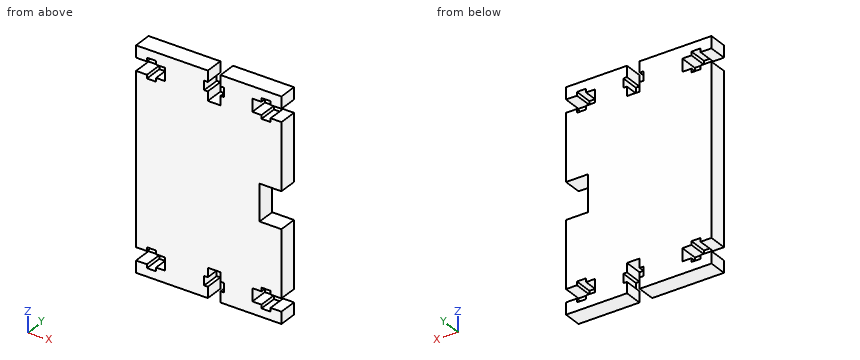
```python
from build123d import *

# Parameters (mm, degrees)
EXTRUDE_1_DEPTH     = 5
CUT_EXTRUDE_1_DEPTH = 5


with BuildPart() as part:
    # 草图1 → 凸台-拉伸1 (new body)
    with BuildSketch(Plane(origin=(0, 0, 0), x_dir=(1, 0, 0), z_dir=(0, 1, 0))):
        Polygon((-19.743275532, 30), (-19.743275532, 26.75), (-16.743275532, 26.75), (-16.743275532, 27.75), (-14.243275532, 27.75), (-14.243275532, 26.75), (-11.743275532, 26.75), (-11.743275532, 23.25), (-14.243275532, 23.25), (-14.243275532, 22.25), (-16.743275532, 22.25), (-16.743275532, 23.25), (-19.743275532, 23.25), (-19.743275532, -23.25), (-16.743275532, -23.25), (-16.743275532, -22.25), (-14.243275532, -22.25), (-14.243275532, -23.25), (-11.743275532, -23.25), (-11.743275532, -26.75), (-14.243275532, -26.75), (-14.243275532, -27.75), (-16.743275532, -27.75), (-16.743275532, -26.75), (-19.743275532, -26.75), (-19.743275532, -30), (20.256724468, -30), (20.256724468, -26.75), (17.256724468, -26.75), (17.256724468, -27.75), (14.756724468, -27.75), (14.756724468, -26.75), (12.256724468, -26.75), (12.256724468, -23.25), (14.756724468, -23.25), (14.756724468, -22.25), (17.256724468, -22.25), (17.256724468, -23.25), (20.256724468, -23.25), (20.256724468, -5), (14.256724468, -5), (14.256724468, 5), (20.256724468, 5), (20.256724468, 23.25), (17.256724468, 23.25), (17.256724468, 22.25), (14.756724468, 22.25), (14.756724468, 23.25), (12.256724468, 23.25), (12.256724468, 26.75), (14.756724468, 26.75), (14.756724468, 27.75), (17.256724468, 27.75), (17.256724468, 26.75), (20.256724468, 26.75), (20.256724468, 30), align=None)
    extrude(amount=EXTRUDE_1_DEPTH)

    # 草图2 → 切除-拉伸1 (cut)
    with BuildSketch(Plane(origin=(0, 5, 0), x_dir=(1, 0, 0), z_dir=(0, 1, 0))):
        Polygon((0, 30), (0, 27), (-1, 27), (-1, 24.5), (0, 24.5), (0, 22), (3.5, 22), (3.5, 24.5), (4.5, 24.5), (4.5, 27), (3.5, 27), (3.5, 30), align=None)
        Polygon((3.5, -30), (0, -30), (0, -27), (-1, -27), (-1, -24.5), (0, -24.5), (0, -22), (3.5, -22), (3.5, -24.5), (4.5, -24.5), (4.5, -27), (3.5, -27), align=None)
    extrude(amount=-CUT_EXTRUDE_1_DEPTH, mode=Mode.SUBTRACT)


solid = part.part
```
Design review of the part built by this model. Coordinates are the model's own, in mm. Give positions to 0.01 mm unless a question says otherwise; leave off trailing zeros. Order: outer loops, then holes, each group sorted by start corner. A loop starts at its lowest first (then second) coordinate and runs counter-clockwise, first axis right, second up. Notation, with made-up numbers: M 89,43.5 L 142,43.5 A15 ccw 142,53.5 Z; hole C 39.5,40 d6. An arc over 180 degrees is marked long. One line per question, with ' | ' between items. Start each with the question number.
Q1. For pin 1 Ø3 at (y, z) = (3, -25) entering from -X; pin 2 Ø0.8 at (y, z) = (3.5, 25) entering from +X, all flat-tipped, find the tip position at first contact; note any pin that passes through.
Q2. We need section A-A (z = 3.5). Write out the cut boundary in (x, y), plus the area to 3 significant figures.
Q3. For L1, parallel to Z at x = -15, y = 2.2; L2, parallel to Z at x = 16, y = 4.55; L3, parallel to X at y = 2.2, z = -23, list the stretches that pass through material, from the lowest coordinate up. Write a range as [from, to].
Returned:
1) pin 1: x = -11.74 | pin 2: x = 12.26
2) outline: M -19.74,0 L 14.26,0 L 14.26,5 L -19.74,5 Z | area: 170 mm2
3) L1: [-30, -27.75], [-22.25, 22.25], [27.75, 30] | L2: [-30, -27.75], [-22.25, -5], [5, 22.25], [27.75, 30] | L3: [-19.74, -16.74], [-14.24, 0], [3.5, 14.76], [17.26, 20.26]
